For this review, use the dimensioned drawing (mm, ordinates from the lowest corner) and the shaded views. Round coordinates to 2 decimals unless told otherwise and drop trailing zeros. Loops run counter-clockwise (first coordinate to the right, second up) from the corner with the lowest first, then second, coordinate; pieces in that order, holes last. Notation, with made-up numbers: (35.25, 74.25) -> (74.25, 74.25) arc R26 cw to (74.25, 92.25) -> close; hole circle Ø3 at (-13, -27.75). An arc over 180 degrees is marked (long way). Write each question's results on one line, items separated by ' | '. Start each with the question number.
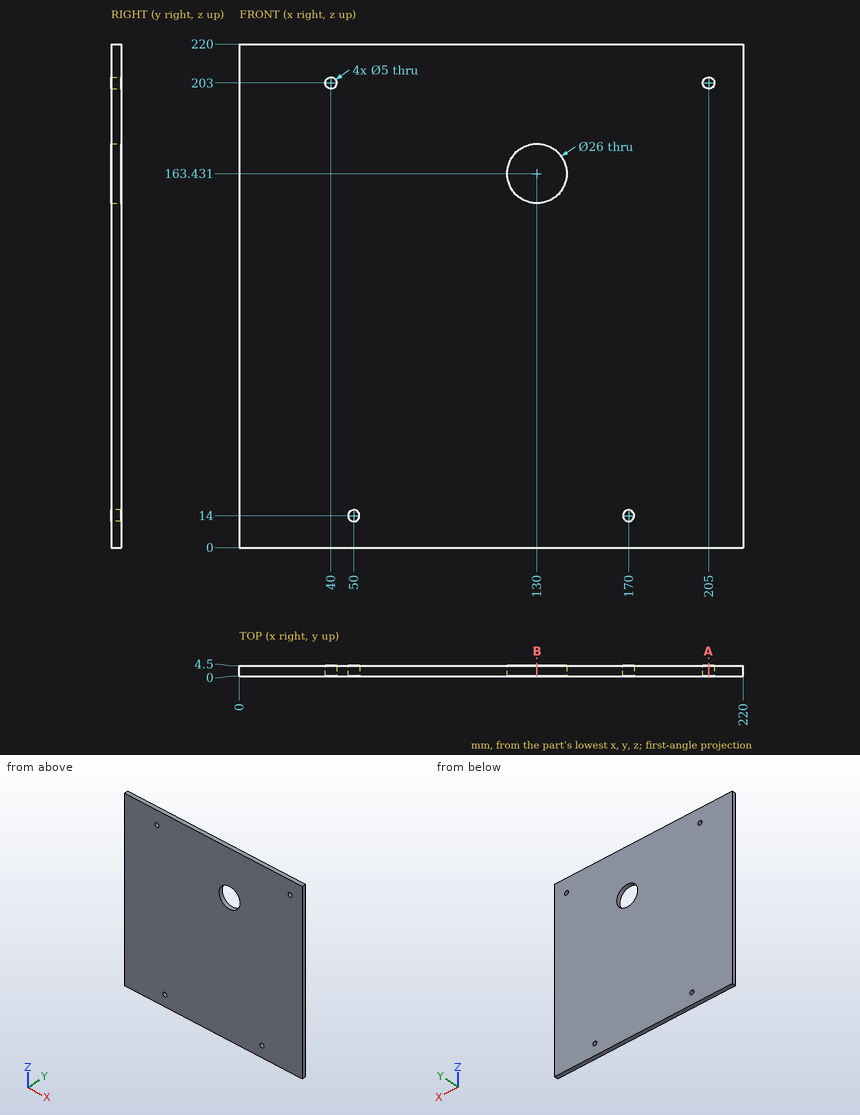
1) Take a section at A-A (x = 205). Write out the cut boundary in (y, z).
2) Take a section at B-B (x = 130). Write out the cut boundary in (y, z), plus the area to 3 significant figures.
3) To check wall thickness, follow line 1 (X direction, y = 2.8, z = 203); line 2 (X direction, y = 1.85, z = 14); line 3 (Z direction, x = 205, y = 1.2). State the ranges of each line that lie inside material, in increasing order. Write a range as from..to.
Geometry check:
1) outline: (0, 0) -> (4.5, 0) -> (4.5, 200.5) -> (0, 200.5) -> close; (0, 205.5) -> (4.5, 205.5) -> (4.5, 220) -> (0, 220) -> close
2) outline: (0, 0) -> (4.5, 0) -> (4.5, 150.43) -> (0, 150.43) -> close; (0, 176.43) -> (4.5, 176.43) -> (4.5, 220) -> (0, 220) -> close | area: 873 mm^2
3) line 1: x = 0..37.5, 42.5..202.5, 207.5..220 | line 2: x = 0..47.5, 52.5..167.5, 172.5..220 | line 3: z = 0..200.5, 205.5..220
